from build123d import *

# Parameters (mm, degrees)
SKETCH2_W           = 9.52
SKETCH2_H           = 28.42
SKETCH2_W_2         = 3.01
SKETCH2_H_2         = 6
BOSS_EXTRUDE1_DEPTH = 10
SKETCH3_R           = 1.96857517
CUT_EXTRUDE1_DEPTH  = 9
FILLET1_R           = 1


with BuildPart() as part:
    # Sketch2 → Boss-Extrude1 (new body)
    with BuildSketch(Plane.XY):
        with BuildLine():
            Line((0, 66.651771766), (0, 33.391771766))
            Line((0, 33.391771766), (-16.03, 33.391771766))
            ThreePointArc((-16.03, 33.391771766), (-16.53, 32.891771766), (-16.03, 32.391771766))
            Line((-16.03, 32.391771766), (1.352234191, 32.391771766))
            Line((1.352234191, 32.391771766), (1.352234191, 34.518218659))
            ThreePointArc((1.352234191, 34.518218659), (1.506462672, 34.749146821), (1.77885672, 34.695149386))
            Line((1.77885672, 34.695149386), (4.496782459, 31.98195805))
            ThreePointArc((4.496782459, 31.98195805), (4.727391952, 30.826554208), (3.747902937, 30.171771766))
            Line((3.747902937, 30.171771766), (-21.54, 30.171771766))
            ThreePointArc((-21.54, 30.171771766), (-22.247106781, 30.464664985), (-22.54, 31.171771766))
            Line((-22.54, 31.171771766), (-22.54, 32.942649485))
            ThreePointArc((-22.54, 32.942649485), (-22.832893219, 33.649756266), (-23.54, 33.942649485))
            Line((-23.54, 33.942649485), (-23.98462025, 33.942649485))
            ThreePointArc((-23.98462025, 33.942649485), (-25.801884678, 34.695385057), (-26.55462025, 36.512649485))
            Line((-26.55462025, 36.512649485), (-26.55462025, 44.391771766))
            ThreePointArc((-26.55462025, 44.391771766), (-25.801884678, 46.209036193), (-23.98462025, 46.961771766))
            Line((-23.98462025, 46.961771766), (-23.54, 46.961771766))
            ThreePointArc((-23.54, 46.961771766), (-22.832893219, 47.254664985), (-22.54, 47.961771766))
            Line((-22.54, 47.961771766), (-22.54, 67.401771766))
            ThreePointArc((-22.54, 67.401771766), (-22.832893219, 68.108878547), (-23.54, 68.401771766))
            Line((-23.54, 68.401771766), (-23.98462025, 68.401771766))
            ThreePointArc((-23.98462025, 68.401771766), (-25.801884678, 69.154507338), (-26.55462025, 70.971771766))
            Line((-26.55462025, 70.971771766), (-26.55462025, 77.401771766))
            Line((-26.55462025, 77.401771766), (-26.55462025, 79.000903717))
            ThreePointArc((-26.55462025, 79.000903717), (-25.801884678, 80.818168145), (-23.98462025, 81.570903717))
            Line((-23.98462025, 81.570903717), (-20.021565093, 81.570903717))
            ThreePointArc((-20.021565093, 81.570903717), (-18.905624991, 81.31597989), (-18.011069886, 80.601781295))
            Line((-18.011069886, 80.601781295), (-17.190935487, 79.571798553))
            ThreePointArc((-17.190935487, 79.571798553), (-12.815621218, 76.078617097), (-7.357501728, 74.831771766))
            Line((-7.357501728, 74.831771766), (0.623852111, 74.831771766))
            ThreePointArc((0.623852111, 74.831771766), (2.441116539, 74.079036193), (3.193852111, 72.261771766))
            Line((3.193852111, 72.261771766), (3.193852111, 64.016682225))
            ThreePointArc((3.193852111, 64.016682225), (2.79053513, 63.543838386), (2.26, 63.867533241))
            Line((2.26, 63.867533241), (1.347357771, 66.651771766))
            Line((1.347357771, 66.651771766), (0, 66.651771766))
        make_face()
        with Locations((-11.27, 54.111771766)):
            Rectangle(SKETCH2_W, SKETCH2_H, mode=Mode.SUBTRACT)
        with Locations((-20.2649024, 75.392647139)):
            Rectangle(SKETCH2_W_2, SKETCH2_H_2, mode=Mode.SUBTRACT)
        with Locations((-20.2649024, 40.392647139)):
            Rectangle(SKETCH2_W_2, SKETCH2_H_2, mode=Mode.SUBTRACT)
    extrude(amount=BOSS_EXTRUDE1_DEPTH)

    # Sketch3 → Cut-Extrude1 (cut)
    with BuildSketch(Plane.ZY.offset(26.55462025)):
        with Locations(Location((5, 40.452210625, 0), (0, 0, 270))):
            Circle(SKETCH3_R)
        with Locations(Location((5, 74.986337741, 0), (0, 0, 270))):
            Circle(SKETCH3_R)
    extrude(amount=-CUT_EXTRUDE1_DEPTH, mode=Mode.SUBTRACT)

    # Fillet1
    fillet1_edges = [part.edges().sort_by_distance(p)[0] for p in [
        (0, 33.391771766, 5),
    ]]
    fillet(fillet1_edges, radius=FILLET1_R)


solid = part.part
Design review of the part built by this model. Coordinates are the model's own, in mm. A direction names the side the tool comes from. Round coordinates to 2 decimals unless told otherwise and drop trailing zeros. Write each loop counter-clockwise with the first axis right and the second up, starting at its lowest first coordinate (ties: lowest second). Pieces come first, ordered by that corner, then holes. Notation, with made-up numbers: (6.5, 70) -> (12.5, 70) arc R22 ccw to (12.5, 83) -> close; hole circle Ø4 at (40, 21.25). An arc over 180 degrees is marked (long way). One line per item, written item: value. Start each with the question number.
Q1. Add section A-A (x = -6). Give the boundary of the cut face in (y, z).
Q2. Add section B-B (z = 8.5). State how many separate pieces and enclosed holes the cut face has, then the cut area to 3 significant figures.
Q3. Insertion check: P1, Ø3, axis at y = 52, z = 7, coming from the +X side; P2, Ø5, axis at x = -10.5, z = 4, coming from the +Y side; P3, Ø5, axis at y = 76, z = 6.5, coming from the +X side. Each pin has a flat end and moves straight along its axis. Give the tip position at first contact, or say it passes through.
Q4. Tool access review of faces 4 (the face through (-22.54, 58, 5)), 5 (the face through (-18.17, 42.42, 5.09)), 6 (the face through (-20, 72.393, 5)): name each direction out of +Z, -Z, +X, -X, +Y, -Y from which nothing blocks a thin tool from reaching the whole face with its end or side.
Q5. To check wall thickness, follow probe 1 along X at (y, z) = (66, 8); probe 2 along X at (y, z) = (64, 3); probe 3 along X at (y, z) = (53, 3.5). State the ranges of each line that lie inside material, in increasing order.
Q6. The part is to be moulded in two halves that separate along X. For faces 1 (the face through (-18.76, 38, 5)), 2 (the face through (-25.782, 34.676, 4.93)), 3 (the face through (-24.2, 42.42, 5.09)), say which applies: pulls with the +X half, pulls with the -X half, needs draft (parallel to the pull), parting line crosses it, or undercut.
Response:
1. outline: (30.17, 0) -> (32.39, 0) -> (32.39, 10) -> (30.17, 10) -> close; (33.39, 0) -> (74.83, 0) -> (74.83, 10) -> (33.39, 10) -> close
2. separate pieces: 1
2. enclosed holes: 3
2. area: 874 mm^2
3. P1: stops at x = 0
3. P2: stops at y = 76.17
3. P3: stops at x = 2.88
4. face 4: +Z, -Z, -X
4. face 5: -X
4. face 6: +Z, -Z
5. probe 1: x = -22.54 to -16.03, -6.51 to 0, 1.56 to 3.19
5. probe 2: x = -22.54 to -16.03, -6.51 to 0, 2.22 to 3.19
5. probe 3: x = -22.54 to -16.03, -6.51 to 0
6. face 1: undercut
6. face 2: pulls with the -X half
6. face 3: needs draft
